For this review, take the finished solid that the model builds, in its own axes (mm). Give positions to 0.01 mm unless a question says otherwise; leave off trailing zeros.
Item 1: For P1, Ø1, axis at x = 13, y = 279, coming from the -Z side, flat-tipped, find the tip position at first contact; note if it passes through.
Item 2: For probe 1 along Y at (x, z) = (2, -7.5); probe 2 along Z at (x, y) = (5, 216.5); probe 3 along Z at (x, y) = (14, 26.5), list the stretches that pass through material, from the lowest coordinate up.
Item 3: Consider section A-A (z = 28). Give the number of separate pieces and of enclosed holes in the cut face, plus the area to 3 significant figures.
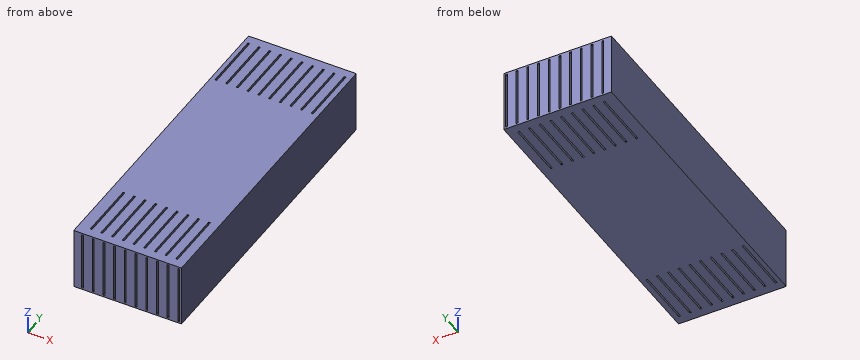
```python
from build123d import *

# Parameters (mm, degrees)
SKETCH1_W           = 120.851681216
SKETCH1_H           = 70
BOSS_EXTRUDE1_DEPTH = 350
SKETCH2_W           = 2
SKETCH2_H           = 66
CUT_EXTRUDE1_DEPTH  = 350
LPATTERN1_COUNT     = 10
LPATTERN1_PITCH     = 12
SKETCH3_W           = 2
SKETCH3_H           = 66
CUT_EXTRUDE2_DEPTH  = 340
LPATTERN2_COUNT     = 10
LPATTERN2_PITCH     = 12
SKETCH4_W           = 2
SKETCH4_H           = 66
CUT_EXTRUDE3_DEPTH  = 340
LPATTERN3_COUNT     = 10
LPATTERN3_PITCH     = 12
SKETCH5_W           = 2
SKETCH5_H           = 66
CUT_EXTRUDE4_DEPTH  = 68
LPATTERN4_COUNT     = 9
LPATTERN4_PITCH     = 12
SKETCH6_W           = 2
SKETCH6_H           = 66
CUT_EXTRUDE5_DEPTH  = 68
LPATTERN5_COUNT     = 9
LPATTERN5_PITCH     = 12
SKETCH7_W           = 2
SKETCH7_H           = 66
CUT_EXTRUDE6_DEPTH  = 68
LPATTERN6_COUNT     = 10
LPATTERN6_PITCH     = 12
SKETCH8_W           = 2
SKETCH8_H           = 66
CUT_EXTRUDE7_DEPTH  = 68
LPATTERN7_COUNT     = 10
LPATTERN7_PITCH     = 12
SKETCH9_W           = 2
SKETCH9_H           = 66
BOSS_EXTRUDE2_DEPTH = 10
LPATTERN9_COUNT     = 10
LPATTERN9_PITCH     = 12
SKETCH11_W          = 2
SKETCH11_H          = 66
BOSS_EXTRUDE4_DEPTH = 10
LPATTERN10_COUNT    = 9
LPATTERN10_PITCH    = 12


with BuildPart() as part:
    # Sketch1 → Boss-Extrude1 (new body)
    with BuildSketch(Plane(origin=(0, 0, 0), x_dir=(1, 0, 0), z_dir=(0, 1, 0))):
        Rectangle(SKETCH1_W, SKETCH1_H)
    extrude(amount=BOSS_EXTRUDE1_DEPTH)

    # Sketch2 → Cut-Extrude1 (cut)
    with BuildSketch(Plane(origin=(0, 350, 0), x_dir=(1, 0, 0), z_dir=(0, 1, 0))):
        with Locations((57.425840608, 0)):
            Rectangle(SKETCH2_W, SKETCH2_H)
    cut_extrude1 = extrude(amount=-CUT_EXTRUDE1_DEPTH, mode=Mode.SUBTRACT)

    # LPattern1: Cut-Extrude1 ×10
    with Locations(*[(-i * LPATTERN1_PITCH, 0, 0) for i in range(1, LPATTERN1_COUNT)]):
        add(cut_extrude1, mode=Mode.SUBTRACT)

    # Sketch3 → Cut-Extrude2 (cut)
    with BuildSketch(Plane(origin=(0, 350, 0), x_dir=(1, 0, 0), z_dir=(0, 1, 0))):
        with Locations((53.425840608, 0)):
            Rectangle(SKETCH3_W, SKETCH3_H)
    cut_extrude2 = extrude(amount=-CUT_EXTRUDE2_DEPTH, mode=Mode.SUBTRACT)

    # LPattern2: Cut-Extrude2 ×10
    with Locations(*[(-i * LPATTERN2_PITCH, 0, 0) for i in range(1, LPATTERN2_COUNT)]):
        add(cut_extrude2, mode=Mode.SUBTRACT)

    # Sketch4 → Cut-Extrude3 (cut)
    with BuildSketch(Plane.XZ):
        with Locations((-46.574159392, 0)):
            Rectangle(SKETCH4_W, SKETCH4_H)
    cut_extrude3 = extrude(amount=-CUT_EXTRUDE3_DEPTH, mode=Mode.SUBTRACT)

    # LPattern3: Cut-Extrude3 ×10
    with Locations(*[(i * LPATTERN3_PITCH, 0, 0) for i in range(1, LPATTERN3_COUNT)]):
        add(cut_extrude3, mode=Mode.SUBTRACT)

    # Sketch5 → Cut-Extrude4 (cut)
    with BuildSketch(Plane(origin=(0, 0, -35), x_dir=(-1, 0, 0), z_dir=(0, 0, -1))):
        with Locations((-49.425840608, 307)):
            Rectangle(SKETCH5_W, SKETCH5_H)
    cut_extrude4 = extrude(amount=-CUT_EXTRUDE4_DEPTH, mode=Mode.SUBTRACT)

    # LPattern4: Cut-Extrude4 ×9
    with Locations(*[(-i * LPATTERN4_PITCH, 0, 0) for i in range(1, LPATTERN4_COUNT)]):
        add(cut_extrude4, mode=Mode.SUBTRACT)

    # Sketch6 → Cut-Extrude5 (cut)
    with BuildSketch(Plane.XY.offset(35)):
        with Locations((49.425840608, 43)):
            Rectangle(SKETCH6_W, SKETCH6_H)
    cut_extrude5 = extrude(amount=-CUT_EXTRUDE5_DEPTH, mode=Mode.SUBTRACT)

    # LPattern5: Cut-Extrude5 ×9
    with Locations(*[(-i * LPATTERN5_PITCH, 0, 0) for i in range(1, LPATTERN5_COUNT)]):
        add(cut_extrude5, mode=Mode.SUBTRACT)

    # Sketch7 → Cut-Extrude6 (cut)
    with BuildSketch(Plane(origin=(0, 0, -35), x_dir=(-1, 0, 0), z_dir=(0, 0, -1))):
        with Locations((-53.425840608, 43)):
            Rectangle(SKETCH7_W, SKETCH7_H)
    cut_extrude6 = extrude(amount=-CUT_EXTRUDE6_DEPTH, mode=Mode.SUBTRACT)

    # LPattern6: Cut-Extrude6 ×10
    with Locations(*[(-i * LPATTERN6_PITCH, 0, 0) for i in range(1, LPATTERN6_COUNT)]):
        add(cut_extrude6, mode=Mode.SUBTRACT)

    # Sketch8 → Cut-Extrude7 (cut)
    with BuildSketch(Plane.XY.offset(35)):
        with Locations((53.425840608, 307)):
            Rectangle(SKETCH8_W, SKETCH8_H)
    cut_extrude7 = extrude(amount=-CUT_EXTRUDE7_DEPTH, mode=Mode.SUBTRACT)

    # LPattern7: Cut-Extrude7 ×10
    with Locations(*[(-i * LPATTERN7_PITCH, 0, 0) for i in range(1, LPATTERN7_COUNT)]):
        add(cut_extrude7, mode=Mode.SUBTRACT)


with BuildPart() as body_2:
    # Sketch9 → Boss-Extrude2 (new body)
    with BuildSketch(Plane(origin=(0, 350, 0), x_dir=(1, 0, 0), z_dir=(0, 1, 0))):
        with Locations((53.425840608, 0)):
            Rectangle(SKETCH9_W, SKETCH9_H)
    boss_extrude2 = extrude(amount=-BOSS_EXTRUDE2_DEPTH)


with BuildPart() as lpattern9_1:
    # LPattern9: pattern copy
    add(boss_extrude2.moved(Location(Vector(-1, 0, 0) * (1 * LPATTERN9_PITCH))))


with BuildPart() as lpattern9_2:
    # LPattern9: pattern copy
    add(boss_extrude2.moved(Location(Vector(-1, 0, 0) * (2 * LPATTERN9_PITCH))))


with BuildPart() as lpattern9_3:
    # LPattern9: pattern copy
    add(boss_extrude2.moved(Location(Vector(-1, 0, 0) * (3 * LPATTERN9_PITCH))))


with BuildPart() as lpattern9_4:
    # LPattern9: pattern copy
    add(boss_extrude2.moved(Location(Vector(-1, 0, 0) * (4 * LPATTERN9_PITCH))))


with BuildPart() as lpattern9_5:
    # LPattern9: pattern copy
    add(boss_extrude2.moved(Location(Vector(-1, 0, 0) * (5 * LPATTERN9_PITCH))))


with BuildPart() as lpattern9_6:
    # LPattern9: pattern copy
    add(boss_extrude2.moved(Location(Vector(-1, 0, 0) * (6 * LPATTERN9_PITCH))))


with BuildPart() as lpattern9_7:
    # LPattern9: pattern copy
    add(boss_extrude2.moved(Location(Vector(-1, 0, 0) * (7 * LPATTERN9_PITCH))))


with BuildPart() as lpattern9_8:
    # LPattern9: pattern copy
    add(boss_extrude2.moved(Location(Vector(-1, 0, 0) * (8 * LPATTERN9_PITCH))))


with BuildPart() as lpattern9_9:
    # LPattern9: pattern copy
    add(boss_extrude2.moved(Location(Vector(-1, 0, 0) * (9 * LPATTERN9_PITCH))))


with BuildPart() as part_1:
    add(part.part)

    # Combine2: union LPattern9_1, LPattern9_2, LPattern9_3, LPattern9_4, LPattern9_5, LPattern9_6, LPattern9_7, LPattern9_8, LPattern9_9, body 2
    add(lpattern9_1.part)
    add(lpattern9_2.part)
    add(lpattern9_3.part)
    add(lpattern9_4.part)
    add(lpattern9_5.part)
    add(lpattern9_6.part)
    add(lpattern9_7.part)
    add(lpattern9_8.part)
    add(lpattern9_9.part)
    add(body_2.part)

    # Sketch11 → Boss-Extrude4 (add)
    with BuildSketch(Plane.XZ):
        with Locations((49.425840608, 0)):
            Rectangle(SKETCH11_W, SKETCH11_H)
    boss_extrude4 = extrude(amount=-BOSS_EXTRUDE4_DEPTH)

    # LPattern10: Boss-Extrude4 ×9
    with Locations(*[(-i * LPATTERN10_PITCH, 0, 0) for i in range(1, LPATTERN10_COUNT)]):
        add(boss_extrude4)


solid = part_1.part
```
Resolved:
1. P1: stops at z = 33
2. probe 1: y = 0 to 10, 340 to 350
2. probe 2: z = -35 to -33, 33 to 35
2. probe 3: z = -35 to -33
3. separate pieces: 11
3. enclosed holes: 19
3. area: 22,800 mm2
